Geometry: final body of the model. Coordinates: model frame, mm. Face numbers are marked on the shaded views. A direction names the side the tool comes from. Coordinates: 2 decimals unless noted, no trailing zeros. Order: outer loops, then holes, each group sorted by start corner. A loop starts at its lowest first (then second) coordinate and runs counter-clockwise, first axis right, second up. Notation, with made-up numbers: M -28,46.25 L 29,46.25 A25 ccw 29,60.25 Z; hole C -25,48 d3. An arc over 180 degrees is marked long. Use CSV: the item, a comma, the result in double quotes. Start each with the question number.
Q1. Section query C-C, the plane z = -4. Output: boundary loops of the cut face in (x, y), and give its area (3 significant figures).
Q2. Section query A-A, the plane z = -11.25. Output: boundary loops of the cut face in (x, y).
Q3. Mould query, pull axis Z, two halves, no side actions, for the marked faces 1, 2, 3 and 4. Classes: +Z half, -Z half, draft (parallel to the pull), parting line (faces both ways), or undercut.
Q4. Section query D-D, the plane x = -10. Output: boundary loops of the cut face in (y, z), and give its area (3 significant figures).
Q5. Section query B-B, the plane x = 0. Output: boundary loops of the cut face in (y, z), and give its area (3 significant figures).
Q6. First-contact query: P1, Ø5, axis at y = 39.5, z = -40, coming from the -X side; P2, Ø3, axis at y = 8.5, z = -39, coming from the +X side; P3, Ø4, axis at x = -2, y = 23.5, coming from the -Z side. Flat tips, straight axial feed; report the tip coordinate or a pass-through.
Q7. Access query for the marked faces 5 and 6. Directions: +Z, -Z, +X, -X, +Y, -Y. A direction counts if a zero-diameter tool reaches every point of the face in a straight line with its end or side. Return the directions, or none.
Q8. Ray query, probe 1 along Y at (x, z) = (-4.5, -19); probe 2 along Y at (x, z) = (-1.25, -19.5); probe 3 along Z at (x, y) = (5, 31). Return the intervals inside material, ascending.
from build123d import *

# Parameters (mm, degrees)
SKETCH1_R           = 1.7
BOSS_EXTRUDE1_DEPTH = 45
CUT_EXTRUDE1_REACH  = 24
SKETCH2_R           = 5.08
SKETCH2_R_2         = 1
FILLET1_R           = 0.5
CUT_EXTRUDE2_DEPTH  = 2
CUT_EXTRUDE3_START  = 17
CUT_EXTRUDE3_DEPTH  = 2


with BuildPart() as part:
    # Sketch1 → Boss-Extrude1 (new body)
    with BuildSketch(Plane(origin=(0, 0, 0), x_dir=(1, 0, 0), z_dir=(0, 1, 0))):
        with BuildLine():
            ThreePointArc((-14.5, 36), (-7.570903506, 40.629874257), (-9.196699141, 48.803300859))
            Line((-9.196699141, 48.803300859), (7.5, 32.106601718))
            Line((7.5, 32.106601718), (7.5, -5))
            Line((7.5, -5), (-7.5, -5))
            Line((-7.5, -5), (-7.5, 29))
            Line((-7.5, 29), (-14.5, 36))
        make_face()
        Circle(SKETCH1_R, mode=Mode.SUBTRACT)
        with Locations((0, 22.5)):
            Circle(SKETCH1_R, mode=Mode.SUBTRACT)
    extrude(amount=BOSS_EXTRUDE1_DEPTH)

    # Sketch2 → Cut-Extrude1 (cut, up to next)
    with BuildSketch(Plane(origin=(7.5, 0, 0), x_dir=(0, 0, -1), z_dir=(1, 0, 0)), mode=Mode.PRIVATE) as cut_extrude1_sk1:
        with Locations((11.25, 22.5)):
            Circle(SKETCH2_R)
    cut_extrude1_tool1 = extrude(cut_extrude1_sk1.sketch, amount=-CUT_EXTRUDE1_REACH, mode=Mode.PRIVATE) & part.part
    add(cut_extrude1_tool1.solids().sort_by_distance((7.5, 22.5, -11.25))[0], mode=Mode.SUBTRACT)
    # Sketch2 → Cut-Extrude1 (cut, up to next)
    with BuildSketch(Plane(origin=(7.5, 0, 0), x_dir=(0, 0, -1), z_dir=(1, 0, 0)), mode=Mode.PRIVATE) as cut_extrude1_sk2:
        with Locations((3.617, 30.133)):
            Circle(SKETCH2_R_2)
    cut_extrude1_tool2 = extrude(cut_extrude1_sk2.sketch, amount=-CUT_EXTRUDE1_REACH, mode=Mode.PRIVATE) & part.part
    add(cut_extrude1_tool2.solids().sort_by_distance((7.5, 30.133, -3.617))[0], mode=Mode.SUBTRACT)
    # Sketch2 → Cut-Extrude1 (cut, up to next)
    with BuildSketch(Plane(origin=(7.5, 0, 0), x_dir=(0, 0, -1), z_dir=(1, 0, 0)), mode=Mode.PRIVATE) as cut_extrude1_sk3:
        with Locations((18.883, 30.133)):
            Circle(SKETCH2_R_2)
    cut_extrude1_tool3 = extrude(cut_extrude1_sk3.sketch, amount=-CUT_EXTRUDE1_REACH, mode=Mode.PRIVATE) & part.part
    add(cut_extrude1_tool3.solids().sort_by_distance((7.5, 30.133, -18.883))[0], mode=Mode.SUBTRACT)
    # Sketch2 → Cut-Extrude1 (cut, up to next)
    with BuildSketch(Plane(origin=(7.5, 0, 0), x_dir=(0, 0, -1), z_dir=(1, 0, 0)), mode=Mode.PRIVATE) as cut_extrude1_sk4:
        with Locations((18.883, 14.867)):
            Circle(SKETCH2_R_2)
    cut_extrude1_tool4 = extrude(cut_extrude1_sk4.sketch, amount=-CUT_EXTRUDE1_REACH, mode=Mode.PRIVATE) & part.part
    add(cut_extrude1_tool4.solids().sort_by_distance((7.5, 14.867, -18.883))[0], mode=Mode.SUBTRACT)
    # Sketch2 → Cut-Extrude1 (cut, up to next)
    with BuildSketch(Plane(origin=(7.5, 0, 0), x_dir=(0, 0, -1), z_dir=(1, 0, 0)), mode=Mode.PRIVATE) as cut_extrude1_sk5:
        with Locations((3.617, 14.867)):
            Circle(SKETCH2_R_2)
    cut_extrude1_tool5 = extrude(cut_extrude1_sk5.sketch, amount=-CUT_EXTRUDE1_REACH, mode=Mode.PRIVATE) & part.part
    add(cut_extrude1_tool5.solids().sort_by_distance((7.5, 14.867, -3.617))[0], mode=Mode.SUBTRACT)

    # Fillet1
    fillet1_edges = [part.edges().sort_by_distance(p)[0] for p in [
        (-9.196699141, 22.5, -48.803300859),
        (-14.5, 22.5, -36),
    ]]
    fillet(fillet1_edges, radius=FILLET1_R)

    # Sketch3 → Cut-Extrude2 (cut, symmetric)
    with BuildSketch(Plane(origin=(0, 22.5, 0), x_dir=(1, 0, 0), z_dir=(0, 1, 0))):
        with BuildLine():
            Line((-8.136038969, 37.136038969), (-2.83273811, 42.439339828))
            Line((-2.83273811, 42.439339828), (-1.772077939, 41.378679656))
            Line((-1.772077939, 41.378679656), (-7.075378798, 36.075378798))
            ThreePointArc((-7.075378798, 36.075378798), (-9.276718417, 34.391359623), (-11.841997191, 33.341997191))
            Line((-11.841997191, 33.341997191), (-13.10825905, 34.60825905))
            ThreePointArc((-13.10825905, 34.60825905), (-10.421379383, 35.477229041), (-8.136038969, 37.136038969))
        make_face()
    extrude(amount=CUT_EXTRUDE2_DEPTH, both=True, mode=Mode.SUBTRACT)

    # Sketch3_2 → Cut-Extrude3 (cut, symmetric)
    with BuildSketch(Plane(origin=(0, 22.5, 0), x_dir=(1, 0, 0), z_dir=(0, 1, 0)).offset(CUT_EXTRUDE3_START)):
        with BuildLine():
            Line((-8.136038969, 37.136038969), (-2.83273811, 42.439339828))
            Line((-2.83273811, 42.439339828), (-1.772077939, 41.378679656))
            Line((-1.772077939, 41.378679656), (-7.075378798, 36.075378798))
            ThreePointArc((-7.075378798, 36.075378798), (-9.276718417, 34.391359623), (-11.841997191, 33.341997191))
            Line((-11.841997191, 33.341997191), (-13.10825905, 34.60825905))
            ThreePointArc((-13.10825905, 34.60825905), (-10.421379383, 35.477229041), (-8.136038969, 37.136038969))
        make_face()
    cut_extrude3 = extrude(amount=CUT_EXTRUDE3_DEPTH, both=True, mode=Mode.SUBTRACT)

    # Mirror1: Cut-Extrude3 across plane
    add(cut_extrude3.mirror(Plane.ZX.offset(22.5)), mode=Mode.SUBTRACT)


solid = part.part
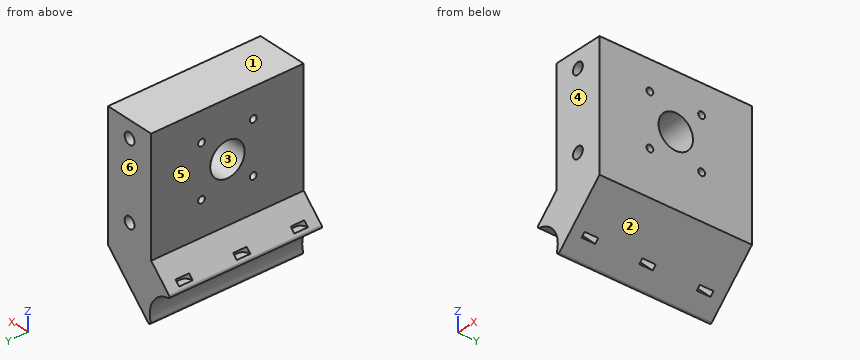
Responses:
1,outline,"M -7.5,0 L 7.5,0 L 7.5,13.94 L -7.5,13.94 Z; M -7.5,15.79 L 7.5,15.79 L 7.5,29.21 L -7.5,29.21 Z; M -7.5,31.06 L 7.5,31.06 L 7.5,45 L -7.5,45 Z"
1,area,"620 mm²"
2,outline,"M -7.5,0 L 7.5,0 L 7.5,17.42 L -7.5,17.42 Z; M -7.5,27.58 L 7.5,27.58 L 7.5,45 L -7.5,45 Z"
3,face 1,"+Z half"
3,face 2,"-Z half"
3,face 3,"undercut"
3,face 4,"draft"
4,outline,"M 0,-37.5 L 45,-37.5 L 45,-31.5 L 0,-31.5 Z; hole M 3.5,-35.71 L 7.5,-35.71 L 7.5,-34.01 L 3.5,-34.01 Z; hole M 20.5,-35.71 L 24.5,-35.71 L 24.5,-34.01 L 20.5,-34.01 Z; hole M 37.5,-35.71 L 41.5,-35.71 L 41.5,-34.01 L 37.5,-34.01 Z"
4,area,"250 mm²"
5,outline,"M 0,-39.61 L 45,-39.61 L 45,-24.2 L 0,-24.2 Z; M 0,-20.8 L 45,-20.8 L 45,-1.7 L 0,-1.7 Z; M 0,1.7 L 45,1.7 L 45,5 L 0,5 Z; hole C 14.87,-18.88 d2; hole C 14.87,-3.62 d2; hole C 22.5,-11.25 d10.16; hole C 30.13,-18.88 d2; hole C 30.13,-3.62 d2"
5,area,"1,610 mm²"
6,P1,"stops at x = -10"
6,P2,"stops at x = 2.11"
6,P3,"stops at z = -43.61"
7,face 5,"+Z, -X, +Y, -Y"
7,face 6,"+Z, -Z, +X, -X, +Y"
8,probe 1,"y = 0 to 13.87, 15.86 to 29.14, 31.13 to 45"
8,probe 2,"y = 0 to 14.08, 15.65 to 29.35, 30.92 to 45"
8,probe 3,"z = -34.61 to -19.38, -18.38 to -4.12, -3.12 to 5"
